Check sheet for the modelled part. Datum: model origin and axes. Units: mm. Face numbers are marked on the shaded views. A direction names the side the tool comes from. Coordinates: 2 decimals unless noted, no trailing zeros. Write each loop counter-clockwise with the first axis right and the second up, starting at its lowest first coordinate (ties: lowest second). Pieces come first, ordered by that corner, then holes. Notation, with made-up numbers: (-30.75, -8.5) -> (-4.75, -8.5) arc R14 cw to (-4.75, 17.5) -> close; hole circle Ø3 at (58, 18.25). An arc over 180 degrees is marked (long way). One line per item, written item: value. Start each with the question number.
1) Sectioned sample at C-C on x = 2.5. Enter the section's corners in (y, z), plus the area to 3 significant figures.
2) Sectioned sample at A-A on z = 0. Enter the section's corners in (x, y).
3) Draft check along Z on the marked faces 4, 5 and 6. Enter one of: +Z half, -Z half, draft (parallel to the pull), parting line (faces both ways), or undercut.
4) Scan lines: line 1 along Z through (x, y) = (1.05, -1.75); line 2 along Y through (x, z) = (0.85, 0); line 3 along Z through (x, y) = (1.6, -2). Record each from-to range of solid material in increasing order. Write a range as [from, to].
5) Set-up check for the marked faces 1, 2 and 3: record each of +Z, -Z, +X, -X, +Y, -Y from which the full face is reachable in a straight line by a thin tool's end or side.
6) Sectioned sample at B-B on y = -1. Enter the section's corners in (x, z), plus the area to 3 significant figures.
7) Gauge pin test, flat ends, axial feed: P1, Ø1.5, axis at x = 2.5, z = -1, coming from the +Y side; P2, Ø2, axis at y = 0, z = 0, coming from the -X side; P3, Ø0.9, axis at x = 1, z = -6, coming from the +Y side; P4, Ø1.5, axis at x = 1.5, y = 1.5, coming from the +Z side. Record the tip position at first contact, or that the pin passes through.
8) Sectioned sample at D-D on y = 0.5. Enter the section's corners in (x, z).
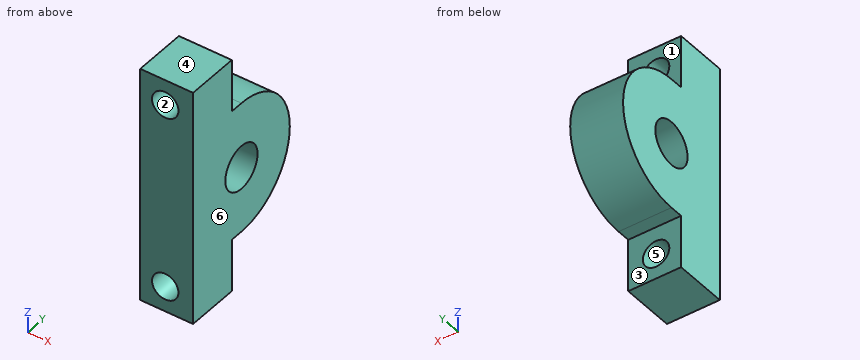
Autodesk Inventor part; units mm, degrees
ref_plane "YZ Plane" through (0, 0, 0) normal (1, 0, 0) x (0, 1, 0)
ref_plane "XZ Plane" through (0, 0, 0) normal (0, 1, 0) x (-1, 0, 0)
ref_plane "XY Plane" through (0, 0, 0) normal (0, 0, 1) x (1, 0, 0)
sketch "Sketch1" plane through (0, 0, 0) normal (1, 0, 0) x (0, 1, 0)
  circle A0 centre (0, 0) radius 1.25
  circle A1 centre (0, 0) radius 3.75
  line L0 (0, -3.75) -> (-3.5355, -3.75)
  line L1 (-3.5355, -3.75) -> (-3.5355, -1.25)
  line L2 (-3.5355, -1.25) -> (0, -1.25)
  line L3 (0, -1.25) -> (0, -3.75)
  line L4 (0, 3.75) -> (-2.9201, 3.75)
  line L5 (-2.9201, 3.75) -> (-2.9201, 1.25)
  line L6 (-2.9201, 1.25) -> (0, 1.25)
  line L7 (0, 1.25) -> (0, 3.75)
  line L8 (-3.75, 0) -> (-1.25, 0)
  line L9 (-1.25, 0) -> (-1.25, -3.75)
  line L10 (-1.25, -3.75) -> (-3.75, -3.75)
  line L11 (-3.75, -3.75) -> (-3.75, 0)
  line L12 (-3.75, 0) -> (-1.25, 0)
  line L13 (-1.25, 0) -> (-1.25, 3.75)
  line L14 (-1.25, 3.75) -> (-3.75, 3.75)
  line L15 (-3.75, 3.75) -> (-3.75, 0)
  line L16 (-3.75, 3.75) -> (-0.75, 3.75)
  line L17 (-0.75, 3.75) -> (-0.75, 6.75)
  line L18 (-0.75, 6.75) -> (-3.75, 6.75)
  line L19 (-3.75, 6.75) -> (-3.75, 3.75)
  line L20 (0, -3.75) -> (-2.9201, -3.75)
  line L21 (-0.75, -3.75) -> (-0.75, -6.75)
  line L22 (-0.75, -6.75) -> (-3.75, -6.75)
  line L23 (-3.75, -6.75) -> (-3.75, -3.75)
  line L24 (-0.75, -6.75) -> (-3.75, -6.75)
  line L25 (-3.75, -6.75) -> (-3.75, -3.75)
  line L26 (-3.75, -3.75) -> (-0.75, -3.75)
  line L27 (-0.75, -3.75) -> (-0.75, -6.75)
  dimension "d0" = 2.5
  dimension "d1" = 7.5
  dimension "d2" = 3
  dimension "d3" = 3
extrude "Extrusion1" add sketch "Sketch1" along normal blind 3
sketch "Sketch2" plane through (3, 0, 0) normal (1, 0, 0) x (0, 0, -1)
  circle A0 centre (0, 0) radius 1.25
  dimension "d6" = 2.5
extrude "Extrusion2" cut sketch "Sketch2" against normal blind 10
sketch "Sketch3" plane through (0, -0.75, 6.75) normal (0, 1, 0) x (1, 0, 0)
  line L0 (0, 0) -> (3, 3.0493)
  line L1 (3, 0) -> (3, 13.5)
  line L2 (0, 6.75) -> (4.6316, 6.75)
  circle A0 centre (1.4195, 1.4429) radius 0.75
  line L3 (0, 13.5) -> (3, 10.4507)
  circle A1 centre (1.4195, 12.0571) radius 0.75
  dimension "d9" = 1.5
extrude "Extrusion3" cut sketch "Sketch3" against normal blind 10
properties part number "attachment"
Answers:
1. outline: (-3.75, -6.75) -> (-0.75, -6.75) -> (-0.75, -3.75) -> (0, -3.75) arc R3.75 ccw to (0, 3.75) -> (-0.75, 3.75) -> (-0.75, 6.75) -> (-3.75, 6.75) -> close; hole circle Ø2.5 at (0, 0)
1. area: 63.3 mm2
2. outline: (0, -3.75) -> (3, -3.75) -> (3, -1.25) -> (0, -1.25) -> close; (0, 1.25) -> (3, 1.25) -> (3, 3.75) -> (0, 3.75) -> close
3. face 4: +Z half
3. face 5: undercut
3. face 6: draft
4. line 1: z = [-6.75, -5.96], [-4.65, 4.65], [5.96, 6.75]
4. line 2: y = [-3.75, -1.25], [1.25, 3.75]
4. line 3: z = [-6.75, -6.04], [-4.58, 4.58], [6.04, 6.75]
5. face 1: +Z, +X, -X, +Y
5. face 2: +Y, -Y
5. face 3: -Z, +X, -X, +Y
6. outline: (0, -6.75) -> (3, -6.75) -> (3, -0.75) -> (0, -0.75) -> close; (0, 0.75) -> (3, 0.75) -> (3, 6.75) -> (0, 6.75) -> close; hole circle Ø1.5 at (1.42, -5.31); hole circle Ø1.5 at (1.42, 5.31)
6. area: 32.5 mm2
7. P1: stops at y = 3.74
7. P2: passes through
7. P3: stops at y = -0.75
7. P4: stops at z = 3.67
8. outline: (0, -3.72) -> (3, -3.72) -> (3, -1.15) -> (0, -1.15) -> close; (0, 1.15) -> (3, 1.15) -> (3, 3.72) -> (0, 3.72) -> close
